from build123d import *

# Parameters (mm, degrees)
SKETCH1_R               = 4.7625
BOSS_EXTRUDE1_DEPTH     = 3.81
SKETCH2_R               = 22.5
BOSS_EXTRUDE2_DEPTH     = 7.62
SKETCH3_R               = 24.08993992
BOSS_EXTRUDE3_DEPTH     = 0.62
SKETCH4_R               = 16.66875
SKETCH4_R_2             = 4.7625
CUT_EXTRUDE1_DEPTH      = 8.62
CUT_EXTRUDE1_DEPTH_BACK = 8.62
SKETCH6_R               = 16.66875
SKETCH6_R_2             = 14.12875
BOSS_EXTRUDE4_DEPTH     = 1.27
CUT_EXTRUDE2_DEPTH      = 2.54
SKETCH8_R               = 0.95
CUT_EXTRUDE3_DEPTH      = 13.7
SKETCH9_R               = 12.7
SKETCH9_R_2             = 4.7625
BOSS_EXTRUDE5_DEPTH     = 6.35
SKETCH10_R              = 15.875
BOSS_EXTRUDE6_DEPTH     = 10.16
SKETCH11_R              = 1.25
CUT_EXTRUDE4_DEPTH      = 1
CUT_EXTRUDE4_DEPTH_BACK = 26.4
SKETCH12_R              = 3.2385
CUT_EXTRUDE5_DEPTH      = 18.78
CUT_EXTRUDE5_DEPTH_BACK = 8.62
SKETCH14_R              = 3.175
CUT_EXTRUDE6_DEPTH      = 23.86
SKETCH15_R              = 6.35
CUT_EXTRUDE7_DEPTH      = 7.62
FILLET1_R               = 0.254


with BuildPart() as part:
    # Sketch1 → Boss-Extrude1 (new body, symmetric)
    with BuildSketch(Plane.XY):
        with BuildLine():
            Line((25.373713394, 1.155278592), (15.858570871, 210.139069198))
            ThreePointArc((15.858570871, 210.139069198), (0, 225.292020078), (-15.858570871, 210.139069198))
            Line((-15.858570871, 210.139069198), (-25.373713394, 1.155278592))
            ThreePointArc((-25.373713394, 1.155278592), (0, -25.4), (25.373713394, 1.155278592))
        make_face()
        with Locations((0, 209.417020078)):
            Circle(SKETCH1_R, mode=Mode.SUBTRACT)
    extrude(amount=BOSS_EXTRUDE1_DEPTH, both=True)

    # Sketch2 → Boss-Extrude2 (add)
    with BuildSketch(Plane.XY.offset(3.81)):
        Circle(SKETCH2_R)
    extrude(amount=BOSS_EXTRUDE2_DEPTH)

    # Sketch3 → Boss-Extrude3 (add)
    with BuildSketch(Plane.XY.offset(3.81)):
        Circle(SKETCH3_R)
    extrude(amount=BOSS_EXTRUDE3_DEPTH)

    # Sketch4 → Cut-Extrude1 (cut, two sides)
    with BuildSketch(Plane.XY.offset(3.81)) as cut_extrude1_sk:
        with Locations((0, 87.91702)):
            Circle(SKETCH4_R)
        with Locations((0, 121.500000078)):
            Circle(SKETCH4_R_2)
    extrude(amount=CUT_EXTRUDE1_DEPTH, mode=Mode.SUBTRACT)
    extrude(cut_extrude1_sk.sketch, amount=-CUT_EXTRUDE1_DEPTH_BACK, mode=Mode.SUBTRACT)

    # Sketch6 → Boss-Extrude4 (add)
    with BuildSketch(Plane.XY.offset(3.81)):
        with Locations((0, 87.91702)):
            Circle(SKETCH6_R)
        with Locations((0, 87.91702)):
            Circle(SKETCH6_R_2, mode=Mode.SUBTRACT)
    extrude(amount=-BOSS_EXTRUDE4_DEPTH)

    # Sketch7 → Cut-Extrude2 (cut)
    with BuildSketch(Plane(origin=(0, 0, -3.81), x_dir=(-1, 0, 0), z_dir=(0, 0, -1))):
        with BuildLine():
            Line((-11.79375, -8.35625), (-11.79375, 8.35625))
            Line((-11.79375, 8.35625), (11.79375, 8.35625))
            Line((11.79375, 8.35625), (11.79375, -8.35625))
            Line((11.79375, -8.35625), (11.79375, -22.495943211))
            ThreePointArc((11.79375, -22.495943211), (0, -25.4), (-11.79375, -22.495943211))
            Line((-11.79375, -22.495943211), (-11.79375, -8.35625))
        make_face()
    extrude(amount=-CUT_EXTRUDE2_DEPTH, mode=Mode.SUBTRACT)

    # Sketch8 → Cut-Extrude3 (cut, through all)
    with BuildSketch(Plane(origin=(0, 0, -1.27), x_dir=(-1, 0, 0), z_dir=(0, 0, -1))):
        with Locations((9, -5.5625)):
            Circle(SKETCH8_R)
        with Locations((-9, -5.5625)):
            Circle(SKETCH8_R)
        with Locations((-9, 5.5625)):
            Circle(SKETCH8_R)
        with Locations((9, 5.5625)):
            Circle(SKETCH8_R)
    extrude(amount=-CUT_EXTRUDE3_DEPTH, mode=Mode.SUBTRACT)

    # Sketch9 → Boss-Extrude5 (add)
    with BuildSketch(Plane.XY.offset(3.81)):
        with Locations((0, 209.417020078)):
            Circle(SKETCH9_R)
        with Locations((0, 209.417020078)):
            Circle(SKETCH9_R_2, mode=Mode.SUBTRACT)
    extrude(amount=BOSS_EXTRUDE5_DEPTH)

    # Sketch10 → Boss-Extrude6 (add)
    with BuildSketch(Plane.XY.offset(11.43)):
        Circle(SKETCH10_R)
    extrude(amount=BOSS_EXTRUDE6_DEPTH)

    # Sketch11 → Cut-Extrude4 (cut, two sides)
    with BuildSketch(Plane(origin=(0, 0, -3.81), x_dir=(-1, 0, 0), z_dir=(0, 0, -1))) as cut_extrude4_sk:
        with Locations((-20.743073922, 11.982962866)):
            Circle(SKETCH11_R)
        with Locations((-19.061789704, 0)):
            Circle(SKETCH11_R)
        with Locations((-15.221171432, -11.474657597)):
            Circle(SKETCH11_R)
        with Locations((15.221171432, -11.474657597)):
            Circle(SKETCH11_R)
        with Locations((19.061789704, 0)):
            Circle(SKETCH11_R)
        with Locations((20.743073922, 11.982962866)):
            Circle(SKETCH11_R)
    extrude(amount=CUT_EXTRUDE4_DEPTH, mode=Mode.SUBTRACT)
    extrude(cut_extrude4_sk.sketch, amount=-CUT_EXTRUDE4_DEPTH_BACK, mode=Mode.SUBTRACT)

    # Sketch12 → Cut-Extrude5 (cut, two sides)
    with BuildSketch(Plane.XY.offset(3.81)) as cut_extrude5_sk:
        with Locations((0, 165.458510078)):
            Circle(SKETCH12_R)
    extrude(amount=CUT_EXTRUDE5_DEPTH, mode=Mode.SUBTRACT)
    extrude(cut_extrude5_sk.sketch, amount=-CUT_EXTRUDE5_DEPTH_BACK, mode=Mode.SUBTRACT)

    # Sketch14 → Cut-Extrude6 (cut, through all)
    with BuildSketch(Plane(origin=(0, 0, -1.27), x_dir=(-1, 0, 0), z_dir=(0, 0, -1))):
        Circle(SKETCH14_R)
    extrude(amount=-CUT_EXTRUDE6_DEPTH, mode=Mode.SUBTRACT)

    # Sketch15 → Cut-Extrude7 (cut)
    with BuildSketch(Plane(origin=(0, 0, -1.27), x_dir=(-1, 0, 0), z_dir=(0, 0, -1))):
        Circle(SKETCH15_R)
    extrude(amount=-CUT_EXTRUDE7_DEPTH, mode=Mode.SUBTRACT)

    # Fillet1
    fillet1_edges = [part.edges().sort_by_distance(p)[0] for p in [
        (-22.5, 0, 11.43),
        (-16.66875, 87.91702, -3.81),
        (-16.66875, 87.91702, 2.54),
        (-15.875, 0, 11.43),
    ]]
    fillet(fillet1_edges, radius=FILLET1_R)


solid = part.part
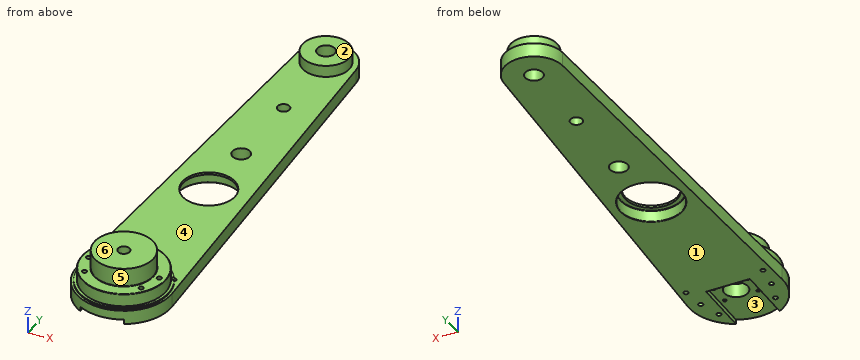
Source: CAD feature listing. Evaluate the final solid. Frame: model axes, mm. Face numbers are marked on the shaded views. A direction names the side the tool comes from. Give positions to 0.01 mm unless a question says otherwise; leave off trailing zeros. Order: outer loops, then holes, each group sorted by start corner. A loop starts at its lowest first (then second) coordinate and runs counter-clockwise, first axis right, second up. Notation, with made-up numbers: (19.25, 21.5) -> (78.25, 21.5) arc R17 cw to (78.25, 30.5) -> close; hole circle Ø3 at (-9, 6.5). An arc over 180 degrees is marked (long way). Write item = value, one per line.
Item 1: Mould query, pull axis Y, two halves, no side actions, for the marked faces 4, 5 and 6. Classes: +Y half, -Y half, draft (parallel to the pull), parting line (faces both ways), or undercut.
Check result:
face_4 = undercut
face_5 = parting line
face_6 = draft
Item 2: Ray query, probe 1 along Y at (x, z) = (0, 4.5); probe 2 along Y at (x, z) = (9, 8.5); probe 3 along Z at (x, y) = (-2.5, 34). Return the intervals inside material, ascending.
Check result:
probe_1 = -22.5 to -6.35, 6.35 to 22.5, 196.72 to 204.65, 214.18 to 222.12
probe_2 = -20.62 to -6.51, -4.61 to 4.61, 6.51 to 20.62, 200.46 to 218.38
probe_3 = -3.81 to 3.81
Item 3: Set-up query: the marked faces 1, 2 and 3. Return all of +Z, -Z, +X, -X, +Y, -Y with unobstructed straight access to the full face (end or side cutting, diameter ignored); none if empty.
Check result:
face_1 = -Z, +X, -X, +Y, -Y
face_2 = +Z, +X, -X, +Y
face_3 = -Z, -Y
Item 4: Section query C-C (y = 31.5). Output: boundary loops of the cut face in (x, z).
Check result:
outline = (-23.99, -3.81) -> (23.99, -3.81) -> (23.99, 3.81) -> (-23.99, 3.81) -> close
Item 5: Section query B-B (x = 0). State how many separate pieces and enclosed holes the cut face has, then the cut area to 3 significant figures.
Check result:
separate_pieces = 6
enclosed_holes = 0
area = 1,960 mm²
Item 6: Contact query for flat-ended pins moving along their axis: pin 1 (11 mm diameter, centred on x = 0, y = 209.42, fed in from -Z); pin 2 (6 mm diameter, centred on x = 0, y = 165.46, fed in from +Z); pin 3 (0.9 mm diameter, centred on x = 9, y = -6, fed in from -Z); pin 4 (2 mm diameter, centred on x = 6, z = -2.5, fed in from -Y). Output: stop coordinate, or through.
Check result:
pin_1 = -3.81
pin_2 = through
pin_3 = 11.43
pin_4 = 8.36
Item 7: Section query A-A (y = 121.5). Output: boundary loops of the cut face in (x, z), then the cut area to 3 significant figures.
Check result:
outline = (-19.89, -3.81) -> (-4.76, -3.81) -> (-4.76, 3.81) -> (-19.89, 3.81) -> close; (4.76, -3.81) -> (19.89, -3.81) -> (19.89, 3.81) -> (4.76, 3.81) -> close
area = 231 mm²
